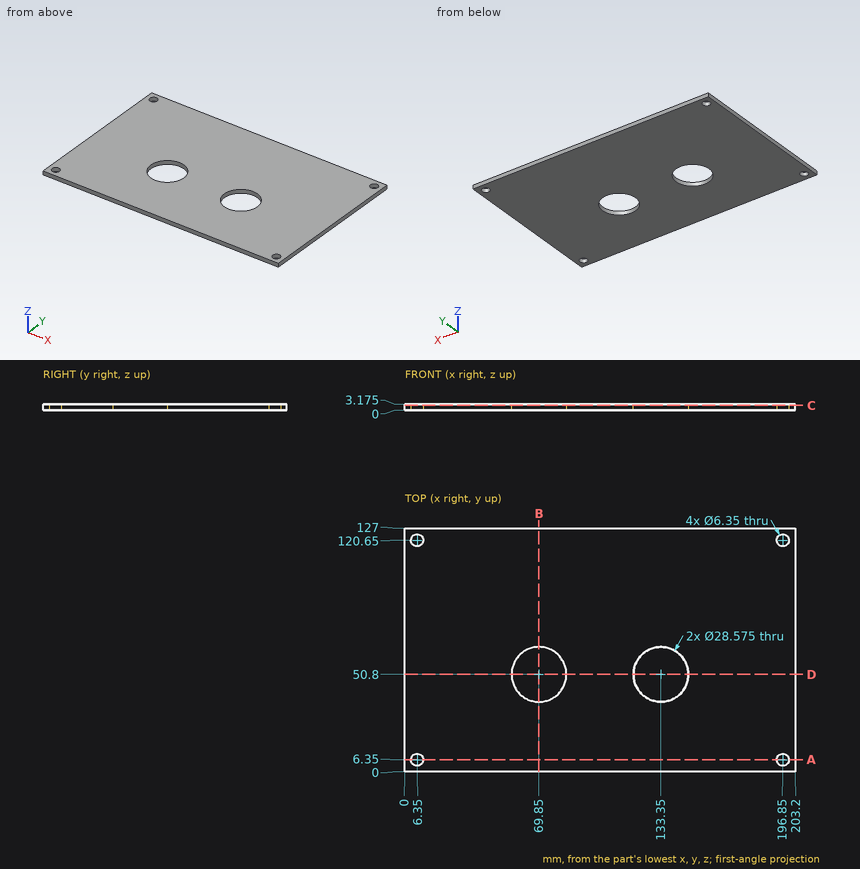
The figure shows three views and two pictorial views of one solid part (mm, origin at its lowest corner). Answer the questions. Coordinates: 2 decimals unless noted, no trailing zeros. Loops run counter-clockwise (first coordinate to the right, second up) from the corner with the lowest first, then second, coordinate; pieces in that order, holes last. Notation, with made-up numbers: (62.5, -2) -> (120.5, -2) arc R18 cw to (120.5, 18) -> close; hole circle Ø3 at (40.5, -26). An arc over 180 degrees is marked (long way). Write item = value, one per line. Start each with the question number.
1) A cutting plane is placed at B-B (x = 69.85). Give the vertices of the cut face in (y, z) (1 decimal), then the cut area to 4 significant figures.
2) A cutting plane is placed at D-D (y = 50.8). Give the vertices of the cut face in (x, z) (1 decimal), then the cut area to 3 significant figures.
3) A cutting plane is placed at A-A (y = 6.35). Give the vertices of the cut face in (x, z) (3 decimals), then the cut area to 3 significant figures.
4) A cutting plane is placed at C-C (z = 2.4). Count the separate pieces of the cut face and the enclosed holes in it, then the cut area to 3 significant figures.
5) Straight lines are drawn through the part: line 1 (X direction, y = 6.35, z = 1.4) (3 decimals); line 2 (Y direction, x = 196.85, z = 2.05) (3 decimals); line 3 (X direction, y = 7.5, z = 0.6). For each, find the intervals that lie inside material, in ascending order. Write a range as from..to.
6) Given pin 1 Ø17 at (x, y) = (133.35, 50.8) entering from +Z, flat-ended and moving along its own axis, determine where the tip first touches the part or whether it passes through.
Responses:
q1.outline = (0, 0) -> (36.5, 0) -> (36.5, 3.2) -> (0, 3.2) -> close; (65.1, 0) -> (127, 0) -> (127, 3.2) -> (65.1, 3.2) -> close
q1.area = 312.5 mm²
q2.outline = (0, 0) -> (55.6, 0) -> (55.6, 3.2) -> (0, 3.2) -> close; (84.1, 0) -> (119.1, 0) -> (119.1, 3.2) -> (84.1, 3.2) -> close; (147.6, 0) -> (203.2, 0) -> (203.2, 3.2) -> (147.6, 3.2) -> close
q2.area = 464 mm²
q3.outline = (0, 0) -> (3.175, 0) -> (3.175, 3.175) -> (0, 3.175) -> close; (9.525, 0) -> (193.675, 0) -> (193.675, 3.175) -> (9.525, 3.175) -> close; (200.025, 0) -> (203.2, 0) -> (203.2, 3.175) -> (200.025, 3.175) -> close
q3.area = 605 mm²
q4.separate_pieces = 1
q4.enclosed_holes = 6
q4.area = 24,400 mm²
q5.line_1 = 0..3.175, 9.525..193.675, 200.025..203.2
q5.line_2 = 0..3.175, 9.525..117.475, 123.825..127
q5.line_3 = 0..3.39, 9.31..193.89, 199.81..203.2
q6.pin_1 = through
